CAD build for the part. Positions are in the model's coordinates, mm. Face numbers are marked on the shaded views. Round coordinates to 2 decimals unless told otherwise and drop trailing zeros. Order: outer loops, then holes, each group sorted by start corner. A loop starts at its lowest first (then second) coordinate and runs counter-clockwise, first axis right, second up. Notation, with made-up numbers: (62.25, 4.5) - (113.25, 4.5) arc R29 cw to (113.25, 30.5) - close; hole circle Ø2 at (0, -6.75). An arc over 180 degrees is marked (long way). Write item = value, one per line.
from build123d import *

# Parameters (mm, degrees)
BOSS_EXTRUDE3_DEPTH = 6.35
SKETCH9_R           = 3.937
CUT_EXTRUDE4_DEPTH  = 127
SKETCH8_W           = 22.86
SKETCH8_H           = 7.62
BOSS_EXTRUDE4_DEPTH = 177.8
CIRPATTERN1_COUNT   = 4
BOSS_EXTRUDE6_DEPTH = 22.86
CIRPATTERN2_COUNT   = 4


with BuildPart() as part:
    # Sketch5 → Boss-Extrude3 (new body)
    with BuildSketch(Plane(origin=(0, 0, 0), x_dir=(1, 0, 0), z_dir=(0, 1, 0))):
        with BuildLine():
            Line((-16.026675419, 11.43), (-132.08, 11.43))
            Line((-132.08, 11.43), (-132.08, -11.43))
            Line((-132.08, -11.43), (-16.026675419, -11.43))
            ThreePointArc((-16.026675419, -11.43), (-13.919396988, -13.919396988), (-11.43, -16.026675419))
            Line((-11.43, -16.026675419), (-11.43, -132.08))
            Line((-11.43, -132.08), (11.43, -132.08))
            Line((11.43, -132.08), (11.43, -16.026675419))
            ThreePointArc((11.43, -16.026675419), (13.919396988, -13.919396988), (16.026675419, -11.43))
            Line((16.026675419, -11.43), (132.08, -11.43))
            Line((132.08, -11.43), (132.08, 11.43))
            Line((132.08, 11.43), (16.026675419, 11.43))
            ThreePointArc((16.026675419, 11.43), (13.919396988, 13.919396988), (11.43, 16.026675419))
            Line((11.43, 16.026675419), (11.43, 132.08))
            Line((11.43, 132.08), (-11.43, 132.08))
            Line((-11.43, 132.08), (-11.43, 16.026675419))
            ThreePointArc((-11.43, 16.026675419), (-13.919396988, 13.919396988), (-16.026675419, 11.43))
        make_face()
    extrude(amount=BOSS_EXTRUDE3_DEPTH)

    # Sketch9 → Cut-Extrude4 (cut)
    with BuildSketch(Plane(origin=(0, 6.35, 0), x_dir=(1, 0, 0), z_dir=(0, 1, 0))):
        Circle(SKETCH9_R)
    extrude(amount=-CUT_EXTRUDE4_DEPTH, mode=Mode.SUBTRACT)

    # Sketch8 → Boss-Extrude4 (add)
    with BuildSketch(Plane(origin=(0, 6.35, 0), x_dir=(1, 0, 0), z_dir=(0, 1, 0))):
        with Locations((0, -128.27)):
            Rectangle(SKETCH8_W, SKETCH8_H)
    boss_extrude4 = extrude(amount=BOSS_EXTRUDE4_DEPTH)

    # CirPattern1: Boss-Extrude4 ×4 about axis
    cirpattern1_axis = Axis((0, 0, 0), (0, 1, 0))
    for i in range(1, CIRPATTERN1_COUNT):
        add(boss_extrude4.rotate(cirpattern1_axis, i * 360 / CIRPATTERN1_COUNT))

    # Sketch13 → Boss-Extrude6 (add)
    with BuildSketch(Plane.XY.offset(11.43)):
        Polygon((-132.08, 184.15), (-137.16, 184.15), (-137.16, 180.34), (-132.08, 165.1), align=None)
    boss_extrude6 = extrude(amount=-BOSS_EXTRUDE6_DEPTH)

    # CirPattern2: Boss-Extrude6 ×4 about axis
    cirpattern2_axis = Axis((0, 0, 0), (0, 1, 0))
    for i in range(1, CIRPATTERN2_COUNT):
        add(boss_extrude6.rotate(cirpattern2_axis, i * 360 / CIRPATTERN2_COUNT))


solid = part.part
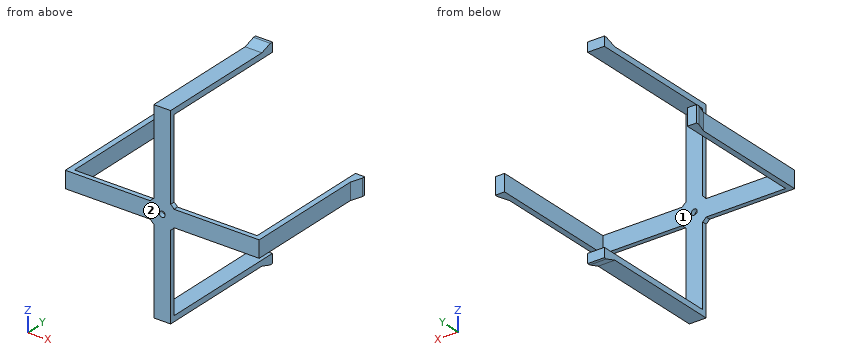
(1) Drop flat-ended pins along their axis: pin 1 (11.5 mm diameter, centred on x = -2, y = 64, fed in from -Z); pin 2 (7 mm diameter, centred on y = 80, z = -2, fed in from +X); pin 3 (4 mm diameter, centred on x = 11.5, z = -12, fed in from -Y); pin 4 (12.5 mm diameter, centred on x = 0, z = 0, fed in from +Y). Give the stop position or say it passes through.
Solved:
pin_1 = -132.08
pin_2 = 132.08
pin_3 = 0
pin_4 = 6.35
(2) Pull direction X, two halves, no side cores. Call the marked faces 1 and 2: released by +X, released by -X, zero draft, split by the parting line, or undercut.
Solved:
face_1 = undercut
face_2 = zero draft
(3) Probe line 1 along X through (y, z) = (2.5, 0); line 2 along Z through (x, y) = (-9, 28). List the from-to ranges inside material, lowest first.
Solved:
line_1 = -132.08 to -3.94, 3.94 to 132.08
line_2 = -132.08 to -124.46, 124.46 to 132.08
(4) Band-saw the part on B-B on y = 132. List the corners of the cut face in (x, z), plus the area to 3 significant figures.
Solved:
outline = (-132.08, -11.43) - (-124.46, -11.43) - (-124.46, 11.43) - (-132.08, 11.43) - close; (-11.43, -132.08) - (11.43, -132.08) - (11.43, -124.46) - (-11.43, -124.46) - close; (-11.43, 124.46) - (11.43, 124.46) - (11.43, 132.08) - (-11.43, 132.08) - close; (124.46, -11.43) - (132.08, -11.43) - (132.08, 11.43) - (124.46, 11.43) - close
area = 697 mm²
(5) Band-saw the part on A-A on x = 0. List the corners of the cut face in (y, z), plus the area to 3 significant figures.
Solved:
outline = (0, -132.08) - (165.1, -132.08) - (180.34, -137.16) - (184.15, -137.16) - (184.15, -124.46) - (6.35, -124.46) - (6.35, -3.94) - (0, -3.94) - close; (0, 3.94) - (6.35, 3.94) - (6.35, 124.46) - (184.15, 124.46) - (184.15, 137.16) - (180.34, 137.16) - (165.1, 132.08) - (0, 132.08) - close
area = 4,450 mm²
(6) Band-saw the part on D-D on z = 53.5. List the corners of the cut face in (x, y), plus the area to 3 significant figures.
Solved:
outline = (-11.43, 0) - (11.43, 0) - (11.43, 6.35) - (-11.43, 6.35) - close
area = 145 mm²
(7) Band-saw the part on C-C on z = 0. List the corners of the cut face in (x, y).
Solved:
outline = (-137.16, 180.34) - (-132.08, 165.1) - (-132.08, 0) - (-3.94, 0) - (-3.94, 6.35) - (-124.46, 6.35) - (-124.46, 184.15) - (-137.16, 184.15) - close; (3.94, 0) - (132.08, 0) - (132.08, 165.1) - (137.16, 180.34) - (137.16, 184.15) - (124.46, 184.15) - (124.46, 6.35) - (3.94, 6.35) - close
